from build123d import *

# Parameters (mm, degrees)
F0_R      = 63.5
F1_DEPTH  = 12.7
F2_R      = 38.1
F3_DEPTH  = 57.15
F4_R      = 50.339294
F5_DEPTH  = 12.7
F6_R      = 5.08
F7_R      = 6.35
F8_DEPTH  = 12.7
F9_W      = 50.8
F9_H      = 50.8
F10_DEPTH = 127


with BuildPart() as f1:
    # F0 (on Top) → F1 (new body)
    with BuildSketch(Plane.XY):
        Circle(F0_R)
    extrude(amount=F1_DEPTH)

    # F2 (on Top) → F3 (join)
    with BuildSketch(Plane.XY):
        Circle(F2_R)
    extrude(amount=F3_DEPTH)

    # F4 (on face) → F5 (join)
    with BuildSketch(Plane.XY.offset(57.15)):
        Circle(F4_R)
    extrude(amount=F5_DEPTH)

    # F6
    f6_edges = [f1.edges().sort_by_distance(p)[0] for p in [
        (-50.339294, 0, 69.85),
    ]]
    fillet(f6_edges, radius=F6_R)

    # F7 (on Top) → F8 (cut)
    with BuildSketch(Plane.XY):
        with Locations((0, 50.170619)):
            Circle(F7_R)
        with Locations((-50.170619, 0)):
            Circle(F7_R)
        with Locations((0, -50.170619)):
            Circle(F7_R)
        with Locations((50.170619, 0)):
            Circle(F7_R)
    extrude(amount=F8_DEPTH, mode=Mode.SUBTRACT)

    # F9 (on Top) → F10 (cut)
    with BuildSketch(Plane.XY):
        Rectangle(F9_W, F9_H)
    extrude(amount=F10_DEPTH, mode=Mode.SUBTRACT)


solid = f1.part
Could you check a few things on this model? Use its own coordinates, in mm. A direction names the side the tool comes from. Coordinates: 2 decimals unless noted, no trailing zeros. Loops run counter-clockwise (first coordinate to the right, second up) from the corner with the lowest first, then second, coordinate; pieces in that order, holes last.
1. Imagine slicing it at C-C (z = 52.5). Please give me the cut outline in (x, y).
2. Imagine slicing it at D-D (z = 9). Please give me the cut outline in (x, y).
3. I need wall thicknesses on L1, parallel to Y at x = 0, z = 5.5; L2, parallel to Z at x = -34, y = 18; L3, parallel to X at y = 9.5, z = 65. Which ranges of each line are inside material? Lowest first, please.
4. Imagine slicing it at A-A (x = 0). Please give me the cut outline in (y, z).
5. For faces 4 (the face through (-10.913, -49.142, 60.907)), 5 (the face through (0, -25.4, 34)), 6 (the face through (-56.514, 0.279, 6.261)), which set-ups out of +Z, -Z, +X, -X, +Y, -Y let a thin tool reach every point of the face, with its end or its side?
6. We'd pull the mould along Y, two halves only. Please class faces 1 (the face through (-1, -30, 69.85)), 2 (the face through (-30.235, -23.183, 34.614)), 3 (the face through (-0.827, -43.875, 6.261)): released by +Y, released by -Y, zero draft, split by the parting line, or undercut.
7. For P1, Ø2, axis at y = -14, z = 28.5, coming from the -X side; P2, Ø12, axis at x = 16, z = 58.5, coming from the -Y side; P3, Ø6, axis at y = -48.5, z = 15, coming from the +X side, each with a flat end and sliding along its axis, tell me the tip position at first contact or that it passes through.
Computed values:
1. outline: circle Ø76.2 at (0, 0); hole (-25.4, -25.4) - (25.4, -25.4) - (25.4, 25.4) - (-25.4, 25.4) - close
2. outline: circle Ø127 at (0, 0); hole circle Ø12.7 at (-50.17, 0); hole (-25.4, -25.4) - (25.4, -25.4) - (25.4, 25.4) - (-25.4, 25.4) - close; hole circle Ø12.7 at (0, -50.17); hole circle Ø12.7 at (0, 50.17); hole circle Ø12.7 at (50.17, 0)
3. L1: y = -63.5 to -56.52, -43.82 to -25.4, 25.4 to 43.82, 56.52 to 63.5
3. L2: z = 0 to 12.7, 57.15 to 69.85
3. L3: x = -49.43 to -25.4, 25.4 to 49.43
4. outline: (-63.5, 0) - (-56.52, 0) - (-56.52, 12.7) - (-63.5, 12.7) - close; (-50.34, 57.15) - (-38.1, 57.15) - (-38.1, 12.7) - (-43.82, 12.7) - (-43.82, 0) - (-25.4, 0) - (-25.4, 69.85) - (-45.26, 69.85) arc R5.08 ccw to (-50.34, 64.77) - close; (25.4, 0) - (43.82, 0) - (43.82, 12.7) - (38.1, 12.7) - (38.1, 57.15) - (50.34, 57.15) - (50.34, 64.77) arc R5.08 ccw to (45.26, 69.85) - (25.4, 69.85) - close; (56.52, 0) - (63.5, 0) - (63.5, 12.7) - (56.52, 12.7) - close
5. face 4: +Z
5. face 5: +Z, -Z
5. face 6: -Z
6. face 1: zero draft
6. face 2: split by the parting line
6. face 3: undercut
7. P1: stops at x = -35.81
7. P2: stops at y = -49.34
7. P3: stops at x = 43.16
